from build123d import *

# Parameters (mm, degrees)
SKETCH1_R               = 100
BOSS_EXTRUDE3_DEPTH     = 90
SKETCH4_W               = 40
SKETCH4_H               = 60
CUT_EXTRUDE2_DEPTH      = 26
CUT_EXTRUDE2_DEPTH_BACK = 12
SKETCH12_R              = 100
BOSS_EXTRUDE4_DEPTH     = 0.1
SKETCH13_R              = 86
CUT_EXTRUDE8_DEPTH      = 80
SKETCH18_R              = 32.5
BOSS_EXTRUDE5_DEPTH     = 25
SKETCH16_R              = 1.6
CUT_EXTRUDE11_DEPTH     = 91.1
SKETCH17_R              = 3
CUT_EXTRUDE12_DEPTH     = 30
SKETCH19_R              = 30
CUT_EXTRUDE13_DEPTH     = 25
SKETCH20_W              = 40
SKETCH20_H              = 5
CUT_EXTRUDE14_DEPTH     = 25
SKETCH21_R              = 1.55
CUT_EXTRUDE15_DEPTH     = 25
SKETCH23_W              = 50
SKETCH23_H              = 15
BOSS_EXTRUDE6_DEPTH     = 3
SKETCH24_W              = 50
SKETCH24_H              = 6
BOSS_EXTRUDE7_DEPTH     = 4
SKETCH25_R              = 1.5
CUT_EXTRUDE17_DEPTH     = 126
BOSS_EXTRUDE8_DEPTH     = 50
SKETCH29_W              = 10
SKETCH29_H              = 11
CUT_EXTRUDE20_DEPTH     = 10
CUT_EXTRUDE21_START     = -10
CUT_EXTRUDE21_DEPTH     = 10
LPATTERN1_COUNT         = 2
LPATTERN1_PITCH         = 20
SKETCH31_R              = 3.881248585
SKETCH31_R_2            = 1.5
BOSS_EXTRUDE9_DEPTH     = 10
SKETCH33_R              = 3.881248585
SKETCH33_R_2            = 1.5
BOSS_EXTRUDE11_DEPTH    = 10
SKETCH34_R              = 3.881248585
SKETCH34_R_2            = 1.5
BOSS_EXTRUDE12_DEPTH    = 10
SKETCH36_R              = 3.881248585
SKETCH36_R_2            = 1.5
CUT_EXTRUDE22_DEPTH     = 10
SKETCH37_R              = 3.881248585
SKETCH37_R_2            = 1.5
CUT_EXTRUDE23_DEPTH     = 10
SKETCH38_W              = 50
SKETCH38_H              = 5
CUT_EXTRUDE24_DEPTH     = 3
SKETCH39_W              = 49.970802014
SKETCH39_H              = 1.005140431
BOSS_EXTRUDE13_DEPTH    = 10
BOSS_EXTRUDE14_REACH    = 203.024
SKETCH40_W              = 49.970802014
SKETCH40_H              = 10
SKETCH41_R              = 12.5
SKETCH41_R_2            = 7.5
BOSS_EXTRUDE15_DEPTH    = 5
CUT_EXTRUDE25_DEPTH     = 37


with BuildPart() as part:
    # Sketch1 → Boss-Extrude3 (new body)
    with BuildSketch(Plane(origin=(0, 0, 0), x_dir=(1, 0, 0), z_dir=(0, 1, 0))):
        Circle(SKETCH1_R)
    extrude(amount=BOSS_EXTRUDE3_DEPTH)

    # Sketch4 → Cut-Extrude2 (cut, two sides)
    with BuildSketch(Plane.XY.offset(105)) as cut_extrude2_sk:
        with Locations((0, 45)):
            Rectangle(SKETCH4_W, SKETCH4_H)
    extrude(amount=CUT_EXTRUDE2_DEPTH, mode=Mode.SUBTRACT)
    extrude(cut_extrude2_sk.sketch, amount=-CUT_EXTRUDE2_DEPTH_BACK, mode=Mode.SUBTRACT)

    # Sketch12 → Boss-Extrude4 (add)
    with BuildSketch(Plane.XZ):
        Circle(SKETCH12_R)
    extrude(amount=BOSS_EXTRUDE4_DEPTH)

    # Sketch13 → Cut-Extrude8 (cut)
    with BuildSketch(Plane(origin=(0, 90, 0), x_dir=(1, 0, 0), z_dir=(0, 1, 0))):
        Circle(SKETCH13_R)
    extrude(amount=-CUT_EXTRUDE8_DEPTH, mode=Mode.SUBTRACT)

    # Sketch18 → Boss-Extrude5 (add)
    with BuildSketch(Plane(origin=(0, 10, 0), x_dir=(1, 0, 0), z_dir=(0, 1, 0))):
        Circle(SKETCH18_R)
    extrude(amount=BOSS_EXTRUDE5_DEPTH)

    # Sketch16 → Cut-Extrude11 (cut, through all)
    with BuildSketch(Plane.XZ.offset(0.1)):
        with Locations((-13, 13)):
            Circle(SKETCH16_R)
        with Locations((13, 13)):
            Circle(SKETCH16_R)
        with Locations((13, -13)):
            Circle(SKETCH16_R)
        with Locations((-13, -13)):
            Circle(SKETCH16_R)
    extrude(amount=-CUT_EXTRUDE11_DEPTH, mode=Mode.SUBTRACT)

    # Sketch17 → Cut-Extrude12 (cut)
    with BuildSketch(Plane.XZ.offset(0.1)):
        with Locations((-13, 13)):
            Circle(SKETCH17_R)
        with Locations((13, 13)):
            Circle(SKETCH17_R)
        with Locations((-13, -13)):
            Circle(SKETCH17_R)
        with Locations((13, -13)):
            Circle(SKETCH17_R)
    extrude(amount=-CUT_EXTRUDE12_DEPTH, mode=Mode.SUBTRACT)

    # Sketch19 → Cut-Extrude13 (cut)
    with BuildSketch(Plane.XZ.offset(0.1)):
        Circle(SKETCH19_R)
    extrude(amount=-CUT_EXTRUDE13_DEPTH, mode=Mode.SUBTRACT)

    # Sketch20 → Cut-Extrude14 (cut)
    with BuildSketch(Plane.XY.offset(93)):
        with Locations((0, 17.5)):
            Rectangle(SKETCH20_W, SKETCH20_H)
    extrude(amount=-CUT_EXTRUDE14_DEPTH, mode=Mode.SUBTRACT)

    # Sketch21 → Cut-Extrude15 (cut)
    with BuildSketch(Plane.XY.offset(93)):
        with Locations((12.45, 67.8)):
            Circle(SKETCH21_R)
        with Locations((-12.45, 67.8)):
            Circle(SKETCH21_R)
        with Locations((-17.05, 30.54)):
            Circle(SKETCH21_R)
        with Locations((17.05, 30.54)):
            Circle(SKETCH21_R)
    extrude(amount=-CUT_EXTRUDE15_DEPTH, mode=Mode.SUBTRACT)

    # Sketch23 → Boss-Extrude6 (add)
    with BuildSketch(Plane(origin=(0, 90, 0), x_dir=(1, 0, 0), z_dir=(0, 1, 0))):
        with Locations((0, 93.523512725)):
            Rectangle(SKETCH23_W, SKETCH23_H)
    extrude(amount=BOSS_EXTRUDE6_DEPTH)

    # Sketch24 → Boss-Extrude7 (add)
    with BuildSketch(Plane(origin=(0, 93, 0), x_dir=(1, 0, 0), z_dir=(0, 1, 0))):
        with Locations((0, 95.023512725)):
            Rectangle(SKETCH24_W, SKETCH24_H)
    extrude(amount=BOSS_EXTRUDE7_DEPTH)

    # Sketch25 → Cut-Extrude17 (cut, through all)
    with BuildSketch(Plane(origin=(25, 0, 0), x_dir=(0, 0, -1), z_dir=(1, 0, 0))):
        with Locations((95.023512725, 95)):
            Circle(SKETCH25_R)
    extrude(amount=-CUT_EXTRUDE17_DEPTH, mode=Mode.SUBTRACT)

    # Sketch27 → Boss-Extrude8 (add)
    with BuildSketch(Plane(origin=(25, 0, 0), x_dir=(0, 0, -1), z_dir=(1, 0, 0))):
        with BuildLine():
            Line((92.023512725, 97), (98.023512725, 97))
            ThreePointArc((98.023512725, 97), (95.023512725, 98.854101966), (92.023512725, 97))
        make_face()
    extrude(amount=-BOSS_EXTRUDE8_DEPTH)

    # Sketch29 → Cut-Extrude20 (cut, through all)
    with BuildSketch(Plane.XY.offset(-92.023512725)):
        with Locations((-10, 98.5)):
            Rectangle(SKETCH29_W, SKETCH29_H)
        with Locations((10, 98.5)):
            Rectangle(SKETCH29_W, SKETCH29_H)
    extrude(amount=-CUT_EXTRUDE20_DEPTH, mode=Mode.SUBTRACT)

    # Sketch30 → Cut-Extrude21 (cut)
    with BuildSketch(Plane(origin=(25, 0, 0), x_dir=(0, 0, -1), z_dir=(1, 0, 0)).offset(CUT_EXTRUDE21_START)):
        with BuildLine():
            Line((92.023512725, 93), (98.023512725, 93))
            ThreePointArc((98.023512725, 93), (95.023512725, 91.890227771), (92.023512725, 93))
        make_face()
    cut_extrude21 = extrude(amount=-CUT_EXTRUDE21_DEPTH, mode=Mode.SUBTRACT)

    # LPattern1: Cut-Extrude21 ×2
    with Locations(*[(-i * LPATTERN1_PITCH, 0, 0) for i in range(1, LPATTERN1_COUNT)]):
        add(cut_extrude21, mode=Mode.SUBTRACT)

    # Sketch31 → Boss-Extrude9 (add)
    with BuildSketch(Plane(origin=(25, 0, 0), x_dir=(0, 0, -1), z_dir=(1, 0, 0))):
        with Locations((95.023512725, 95)):
            Circle(SKETCH31_R)
        with Locations((95.023512725, 95)):
            Circle(SKETCH31_R_2, mode=Mode.SUBTRACT)
    extrude(amount=-BOSS_EXTRUDE9_DEPTH)

    # Sketch33 → Boss-Extrude11 (add)
    with BuildSketch(Plane(origin=(5, 0, 0), x_dir=(0, 0, -1), z_dir=(1, 0, 0))):
        with Locations((95.023512725, 95)):
            Circle(SKETCH33_R)
        with Locations((95.023512725, 95)):
            Circle(SKETCH33_R_2, mode=Mode.SUBTRACT)
    extrude(amount=-BOSS_EXTRUDE11_DEPTH)

    # Sketch34 → Boss-Extrude12 (add)
    with BuildSketch(Plane(origin=(-15, 0, 0), x_dir=(0, 0, -1), z_dir=(1, 0, 0))):
        with Locations((95.023512725, 95)):
            Circle(SKETCH34_R)
        with Locations((95.023512725, 95)):
            Circle(SKETCH34_R_2, mode=Mode.SUBTRACT)
    extrude(amount=-BOSS_EXTRUDE12_DEPTH)

    # Sketch36 → Cut-Extrude22 (cut)
    with BuildSketch(Plane.ZY.offset(-15)):
        with Locations((-97.029162036, 95.048788547)):
            Circle(SKETCH36_R)
        with Locations((-97.029162036, 95.048788547)):
            Circle(SKETCH36_R_2, mode=Mode.SUBTRACT)
    extrude(amount=CUT_EXTRUDE22_DEPTH, mode=Mode.SUBTRACT)

    # Sketch37 → Cut-Extrude23 (cut)
    with BuildSketch(Plane.ZY.offset(5)):
        with Locations((-97.009847138, 94.987072973)):
            Circle(SKETCH37_R)
        with Locations((-97.009847138, 94.987072973)):
            Circle(SKETCH37_R_2, mode=Mode.SUBTRACT)
    extrude(amount=CUT_EXTRUDE23_DEPTH, mode=Mode.SUBTRACT)

    # Sketch38 → Cut-Extrude24 (cut)
    with BuildSketch(Plane(origin=(0, 93, 0), x_dir=(1, 0, 0), z_dir=(0, 1, 0))):
        with Locations((0, 88.523512725)):
            Rectangle(SKETCH38_W, SKETCH38_H)
    extrude(amount=-CUT_EXTRUDE24_DEPTH, mode=Mode.SUBTRACT)

    # Sketch39 → Boss-Extrude13 (add)
    with BuildSketch(Plane(origin=(0, 90, 0), x_dir=(-1, 0, 0), z_dir=(0, -1, 0))):
        with Locations((0.014598993, 100.52094251)):
            Rectangle(SKETCH39_W, SKETCH39_H)
    extrude(amount=BOSS_EXTRUDE13_DEPTH)

    # Sketch40 → Boss-Extrude14 (add, up to next)
    with BuildSketch(Plane(origin=(0, 0, -101.023512725), x_dir=(-1, 0, 0), z_dir=(0, 0, -1)), mode=Mode.PRIVATE) as boss_extrude14_sk1:
        with Locations((0.014598993, 85)):
            Rectangle(SKETCH40_W, SKETCH40_H)
    boss_extrude14_tool1 = extrude(boss_extrude14_sk1.sketch, amount=-BOSS_EXTRUDE14_REACH, mode=Mode.PRIVATE) - part.part
    add(boss_extrude14_tool1.solids().sort_by_distance((-0.014599, 85, -101.023513))[0])

    # Sketch41 → Boss-Extrude15 (add)
    with BuildSketch(Plane(origin=(0, 90, 0), x_dir=(1, 0, 0), z_dir=(0, 1, 0))):
        with Locations((0, -100)):
            Circle(SKETCH41_R)
        with Locations((0, -100)):
            Circle(SKETCH41_R_2, mode=Mode.SUBTRACT)
    extrude(amount=-BOSS_EXTRUDE15_DEPTH)

    # Sketch42 → Cut-Extrude25 (cut)
    with BuildSketch(Plane(origin=(22.204096953, 47.794122581, -296.404157649), x_dir=(1, 0, 0), z_dir=(0, 1, 0))):
        Polygon((-8.101888311, -337.261049447), (12.404969277, -405.762485644), (37.058002756, -394.3841625), (-1.388931435, -334.195344764), align=None)
    extrude(amount=CUT_EXTRUDE25_DEPTH, mode=Mode.SUBTRACT)


solid = part.part
Could you check a few things on this model? Use its own coordinates, in mm. A direction names the side the tool comes from. Coordinates: 2 decimals unless noted, no trailing zeros. Loops run counter-clockwise (first coordinate to the right, second up) from the corner with the lowest first, then second, coordinate; pieces in that order, holes last. Notation, with made-up numbers: (25, -4.75) -> (41, -4.75) arc R26 cw to (41, 17.25) -> close; hole circle Ø9 at (79, -14.5). An arc over 180 degrees is marked (long way). Answer in a Markdown table with one row per item.
(1) Imagine slicing it at D-D (z = 69). List the corners of the cut face in (x, y) for me, plus the area to 3 significant figures.
Results found:
| item | result |
|---|---|
| outline | (-72.38, -0.1) -> (72.38, -0.1) -> (72.38, 90) -> (51.33, 90) -> (51.33, 10) -> (-51.33, 10) -> (-51.33, 90) -> (-72.38, 90) -> close |
| area | 4,830 mm^2 |
(2) Will these pins go through, and if not, where does the flat tip stop? pin 1 Ø1 at (x, z) = (78.5, -33) entering from +Y; pin 2 Ø3.5 at (x, z) = (-13, 13) entering from -Y; pin 3 Ø8 at (y, z) = (65, -78) entering from -X.
Results found:
| item | result |
|---|---|
| pin 1 | stops at y = 10 |
| pin 2 | stops at y = 29.9 |
| pin 3 | stops at x = -67.26 |
(3) Thinking about a two-plate mould opening in Y: for faces 5 (the face through (28.355, 66.035, 88.469)), 6 (the face through (-25, 89, -97)), 7 (the face through (-9.93, 91.185, -97.788)), which applies, released by +Y, released by -Y, zero draft, split by the parting line, or undercut?
Results found:
| item | result |
|---|---|
| face 5 | undercut |
| face 6 | zero draft |
| face 7 | released by +Y |
(4) Imagine slicing it at C-C (y = 56). List the corners of the cut face in (x, z) for me.
Results found:
| item | result |
|---|---|
| outline | (-20, 93) -> (-20, 97.98) arc R100 ccw (long way) to (51.45, 85.75) -> (43.91, 73.95) arc R86 cw (long way) to (26.38, 81.86) -> (30.39, 95.27) arc R100 ccw to (20, 97.98) -> (20, 93) -> close |
(5) Imagine slicing it at A-A (x = 0). Give the number of separate pieces and of enclosed holes in the cut face, plus the area to 3 significant figures.
Results found:
| item | result |
|---|---|
| separate pieces | 3 |
| enclosed holes | 1 |
| area | 4,030 mm^2 |
(6) For faces 1 (the face through (0, 87, -101.024)), 2 (the face through (0, 75, 97)), 3 (the face through (-15, 95, -97)), 4 (the face through (10.6, 27.4, 11.2)), which set-ups out of +Z, -Z, +X, -X, +Y, -Y let a thin tool reach every point of the face, with its end or its side?
Results found:
| item | result |
|---|---|
| face 1 | -Z, +X, -X, +Y, -Y |
| face 2 | +Z |
| face 3 | +Y |
| face 4 | -Y |
(7) Imagine slicing it at B-B (x = 36.5). List the corners of the cut face in (y, z) for me, plus the area to 3 significant figures.
Results found:
| item | result |
|---|---|
| outline | (-0.1, -93.1) -> (90, -93.1) -> (90, -77.87) -> (10, -77.87) -> (10, 77.87) -> (47.79, 77.87) -> (47.79, 93.1) -> (-0.1, 93.1) -> close; (84.79, 77.87) -> (90, 77.87) -> (90, 93.1) -> (84.79, 93.1) -> close |
| area | 3,750 mm^2 |
(8) If I drill on probe 1 along Y at (x, z) = (-12.45, 87); probe 2 along Z at (x, y) = (-23.5, 24.5); probe 3 along Z at (x, y) = (-1, 95), over which ranges is the centre line in solid material (lowest first)?
Results found:
| item | result |
|---|---|
| probe 1 | y = -0.1 to 15, 20 to 66.25, 69.35 to 90 |
| probe 2 | z = -97.2 to -82.73, -22.45 to -18.65, 18.65 to 22.45, 82.73 to 97.2 |
| probe 3 | z = -98.9 to -96.52, -93.52 to -91.14 |
